Check sheet for the modelled part. Datum: model origin and axes. Units: mm. Face numbers are marked on the shaded views. A direction names the side the tool comes from. Give positions to 0.01 mm unless a question says otherwise; leave off trailing zeros. Order: outer loops, then holes, each group sorted by start corner. A loop starts at its lowest first (then second) coordinate and runs counter-clockwise, first axis right, second up. Notation, with made-up numbers: (18, 16.5) -> (43, 16.5) arc R21 ccw to (43, 36.5) -> close; hole circle Ø11 at (20, -25.5). An arc over 180 degrees is marked (long way). Write each question's results on one line, items separated by ' | '.
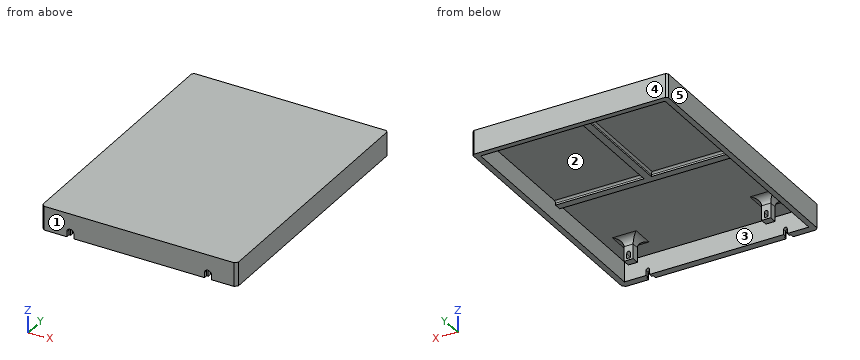
from build123d import *

# Parameters (mm, degrees)
SKETCH1_W           = 100.5
SKETCH1_H           = 134.5
BOSS_EXTRUDE1_DEPTH = 2
SKETCH2_W           = 104.5
SKETCH2_H           = 138.5
SKETCH2_W_2         = 100.5
SKETCH2_H_2         = 134.5
BOSS_EXTRUDE2_DEPTH = 13
BOSS_EXTRUDE3_DEPTH = 2
SKETCH5_W           = 104.5
SKETCH5_H           = 13
BOSS_EXTRUDE4_DEPTH = 2
CUT_EXTRUDE2_DEPTH  = 2
SKETCH8_W           = 5
SKETCH8_H           = 4
BOSS_EXTRUDE5_DEPTH = 12
FILLET1_R           = 4
CUT_EXTRUDE3_DEPTH  = 20
BOSS_EXTRUDE7_DEPTH = 13
CHAMFER1_SIZE       = 1.5
FILLET2_R           = 1


with BuildPart() as part:
    # Sketch1 → Boss-Extrude1 (new body)
    with BuildSketch(Plane.XY):
        with Locations((50.25, -67.25)):
            Rectangle(SKETCH1_W, SKETCH1_H)
    extrude(amount=BOSS_EXTRUDE1_DEPTH)

    # Sketch2 → Boss-Extrude2 (add)
    with BuildSketch(Plane.XY.offset(2)):
        with Locations((50.25, -67.25)):
            Rectangle(SKETCH2_W, SKETCH2_H)
        with Locations((50.25, -67.25)):
            Rectangle(SKETCH2_W_2, SKETCH2_H_2, mode=Mode.SUBTRACT)
    extrude(amount=-BOSS_EXTRUDE2_DEPTH)

    # Sketch3 → Boss-Extrude3 (add)
    with BuildSketch(Plane(origin=(0, 0, 0), x_dir=(-1, 0, 0), z_dir=(0, 0, -1))):
        Polygon((-52.25, 0), (-52.25, -70), (-101.125, -70), (-101.125, -74), (0.625, -74), (0.625, -70), (-48.25, -70), (-48.25, 0), align=None)
    extrude(amount=BOSS_EXTRUDE3_DEPTH)

    # Sketch5 → Boss-Extrude4 (add)
    with BuildSketch(Plane.XZ.offset(136.5)):
        with Locations((50.25, -4.5)):
            Rectangle(SKETCH5_W, SKETCH5_H)
    extrude(amount=BOSS_EXTRUDE4_DEPTH)

    # Sketch4 → Cut-Extrude2 (cut)
    with BuildSketch(Plane.XZ.offset(138.5)):
        with BuildLine():
            Line((89.65, -8.25), (89.65, -11))
            Line((89.65, -11), (85.85, -11))
            Line((85.85, -11), (85.85, -8.25))
            ThreePointArc((85.85, -8.25), (87.75, -6.35), (89.65, -8.25))
        make_face()
        with BuildLine():
            Line((14.65, -8.25), (14.65, -11))
            Line((14.65, -11), (10.85, -11))
            Line((10.85, -11), (10.85, -8.25))
            ThreePointArc((10.85, -8.25), (12.75, -6.35), (14.65, -8.25))
        make_face()
    extrude(amount=-CUT_EXTRUDE2_DEPTH, mode=Mode.SUBTRACT)

    # Sketch8 → Boss-Extrude5 (add)
    with BuildSketch(Plane(origin=(0, 0, 0), x_dir=(-1, 0, 0), z_dir=(0, 0, -1))):
        with Locations((-12.75, -118.5)):
            Rectangle(SKETCH8_W, SKETCH8_H)
        with Locations((-87.75, -118.5)):
            Rectangle(SKETCH8_W, SKETCH8_H)
    extrude(amount=BOSS_EXTRUDE5_DEPTH)

    # Fillet1
    fillet1_edges = [part.edges().sort_by_distance(p)[0] for p in [
        (10.25, -118.5, 0),
        (12.75, -116.5, 0),
        (15.25, -118.5, 0),
        (12.75, -120.5, 0),
        (85.25, -118.5, 0),
        (87.75, -116.5, 0),
        (90.25, -118.5, 0),
        (87.75, -120.5, 0),
    ]]
    fillet(fillet1_edges, radius=FILLET1_R)

    # Sketch7 → Cut-Extrude3 (cut)
    with BuildSketch(Plane.XZ.offset(136.5)):
        with BuildLine():
            Line((88.75, -8.25), (88.75, -11))
            Line((88.75, -11), (86.75, -11))
            Line((86.75, -11), (86.75, -8.25))
            ThreePointArc((86.75, -8.25), (87.75, -7.25), (88.75, -8.25))
        make_face()
        with BuildLine():
            Line((13.75, -8.25), (13.75, -11))
            Line((13.75, -11), (11.75, -11))
            Line((11.75, -11), (11.75, -8.25))
            ThreePointArc((11.75, -8.25), (12.75, -7.25), (13.75, -8.25))
        make_face()
    extrude(amount=-CUT_EXTRUDE3_DEPTH, mode=Mode.SUBTRACT)

    # Sketch13 → Boss-Extrude7 (add)
    with BuildSketch(Plane(origin=(0, 0, -11), x_dir=(-1, 0, 0), z_dir=(0, 0, -1))):
        Polygon((2, -138.5), (3, -138.5), (3, 2), (2, 3), (-102.5, 3), (-103.5, 2), (-103.5, -138.5), (-102.5, -138.5), (-102.5, 2), (2, 2), align=None)
    extrude(amount=-BOSS_EXTRUDE7_DEPTH)

    # Chamfer1
    chamfer1_edges = [part.edges().sort_by_distance(p)[0] for p in [
        (-3, -138.5, -4.5),
        (103.5, -138.5, -4.5),
    ]]
    chamfer(chamfer1_edges, length=CHAMFER1_SIZE)

    # Fillet2
    fillet2_edges = [part.edges().sort_by_distance(p)[0] for p in [
        (76.375, -70, 0),
        (50.25, -74, 0),
        (48.25, -35, 0),
        (24.125, -70, 0),
        (52.25, -35, 0),
    ]]
    fillet(fillet2_edges, radius=FILLET2_R)


solid = part.part
1. Mould release check, pull along Y, two halves, no side actions. Record for the marked faces 3, 4 and 5: +Y half, -Y half, draft (parallel to the pull), parting line (faces both ways), or undercut.
Verdict:
face 3: undercut | face 4: +Y half | face 5: draft
2. Gauge pin test, flat ends, axial feed: pin 1 Ø1.5 at (x, y) = (14.5, -49.5) entering from -Z; pin 2 Ø1.9 at (x, z) = (12.5, -9.5) entering from -Y. Record the tip position at first contact, or that the pin passes through.
Verdict:
pin 1: stops at z = 0 | pin 2: stops at y = -136.5
3. Material ranges on probe 1 along Y at (x, z) = (11.5, -9.75); probe 2 along Y at (x, z) = (86.5, -6.25); probe 3 along Y at (x, z) = (60, -6.5), recorded low to high. Write a range as from..to.
Verdict:
probe 1: y = -136.5..-134.5, -120.5..-116.5, 0..3 | probe 2: y = -138.5..-134.5, -120.5..-116.5, 0..3 | probe 3: y = -138.5..-134.5, 0..3
4. Section check C-C on y = -55. Record the cut outline in (x, z), then the cut area to 3 significant figures.
Verdict:
outline: (-3, -11) -> (0, -11) -> (0, 0) -> (47.25, 0) arc R1 cw to (48.25, -1) -> (48.25, -2) -> (52.25, -2) -> (52.25, -1) arc R1 cw to (53.25, 0) -> (100.5, 0) -> (100.5, -11) -> (103.5, -11) -> (103.5, 2) -> (-3, 2) -> close | area: 287 mm^2
5. Access from +Z, -Z, +X, -X, +Y, -Y to the whole of each face (thin tool, end or side, straight path). Record for the marked faces 1 and 2.
Verdict:
face 1: +Z, -Z, +X, -X, -Y | face 2: -Z
6. Section check B-B on y = -84. Record the cut outline in (x, z), then the cut area to 3 significant figures.
Verdict:
outline: (-3, -11) -> (0, -11) -> (0, 0) -> (100.5, 0) -> (100.5, -11) -> (103.5, -11) -> (103.5, 2) -> (-3, 2) -> close | area: 279 mm^2
7. Section check A-A on x = 79. Record the cut outline in (y, z).
Verdict:
outline: (-138.5, -11) -> (-134.5, -11) -> (-134.5, 0) -> (-75, 0) arc R1 cw to (-74, -1) -> (-74, -2) -> (-70, -2) -> (-70, -1) arc R1 cw to (-69, 0) -> (0, 0) -> (0, -11) -> (3, -11) -> (3, 2) -> (-138.5, 2) -> close
